Verification items for this drawing (mm, ordinates from the low corner). A direction names the side the tool comes from. Round coordinates to 2 decimals unless told otherwise and drop trailing zeros. Order: outer loops, then holes, each group sorted by start corner. A loop starts at its lowest first (then second) coordinate and runs counter-clockwise, first axis right, second up. Notation, with made-up numbers: M 77,-30 L 115,-30 A14 cw 115,-14 Z; hole C -32,60.5 d2. An arc over 180 degrees is marked long. One line per item, written item: value. Start each with the question number.
(1) Cross-section at A-A, the plane x = 7. Enter the section's corners in (y, z), and give its area (3 significant figures).
(2) Depth check by flat-ended pin: pin 1 Ø21 at (y, z) = (25.5, 23) entering from +X; pin 2 Ø10 at (x, z) = (30, 37) entering from +Y; pin 3 Ø1.8 at (y, z) = (3.5, 26) entering from +X; pin 4 Ø5 at (x, z) = (12, 24) entering from +Y. Enter the tip coordinate at first touch or a pass-through.
(3) Access from +Z, -Z, +X, -X, +Y, -Y to the whole of each face (thin tool, end or side, straight path). Record for the marked faces 4, 5, 6, 7 and 8.
(4) Thickness scan on L1, parallel to Z at x = 30, y = 30; L2, parallel to Y at x = 42, z = 22; L3, parallel to X at y = 18, z = 43. Record the ranges inside material, lowest first.
(5) Release check for a two-part mould opening along Z. For the marked faces 1, 2 and 3 record: released by +Z, released by -Z, zero draft, split by the parting line, or undercut.
(6) Cross-section at D-D, the plane x = 42. Enter the section's corners in (y, z), and give its area (3 significant figures).
(7) Cross-section at C-C, the plane z = 14. Enter the section's corners in (x, y).
(8) Cross-section at B-B, the plane y = 38.5. Enter the section's corners in (x, z).
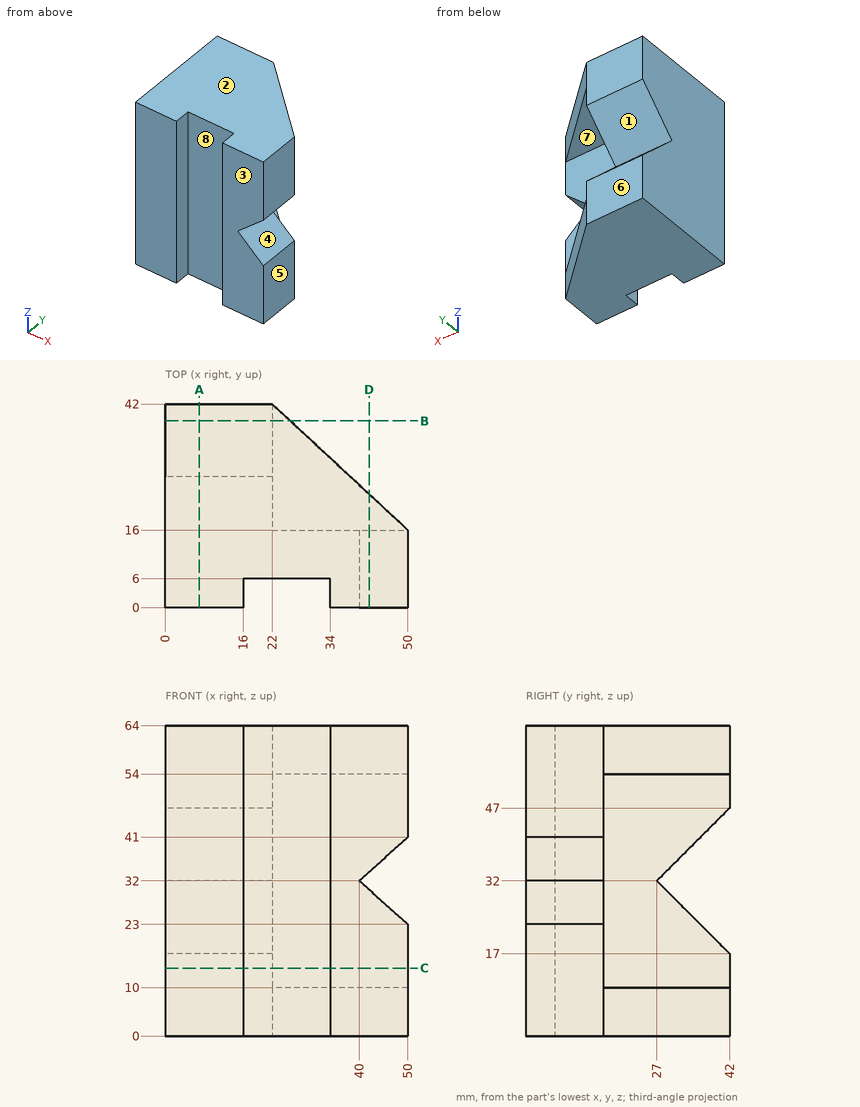
Values found:
1. outline: M 0,0 L 42,0 L 42,17 L 27,32 L 42,47 L 42,64 L 0,64 Z
1. area: 2,460 mm^2
2. pin 1: x = 50
2. pin 2: y = 16
2. pin 3: x = 47.67
2. pin 4: y = 37.5
3. face 4: +X, +Y, -Y
3. face 5: +Z, -Z, +X, +Y, -Y
3. face 6: +Z, -Z, +X, -X, +Y
3. face 7: +X, +Y
3. face 8: +Z, -Z, -Y
4. L1: 0 to 10, 54 to 64
4. L2: 0 to 16
4. L3: 0 to 22
5. face 1: undercut
5. face 2: released by +Z
5. face 3: zero draft
6. outline: M 0,0 L 23.43,0 L 23.43,10 L 16,10 L 16,30.2 L 0,30.2 Z; M 0,33.8 L 16,33.8 L 16,54 L 23.43,54 L 23.43,64 L 0,64 Z
6. area: 1,110 mm^2
7. outline: M 0,0 L 16,0 L 16,6 L 34,6 L 34,0 L 50,0 L 50,16 L 22,16 L 22,42 L 0,42 Z
8. outline: M 0,0 L 25.77,0 L 25.77,10 L 22,10 L 22,20.5 L 0,20.5 Z; M 0,43.5 L 22,43.5 L 22,54 L 25.77,54 L 25.77,64 L 0,64 Z
